from build123d import *

# Parameters (mm, degrees)
SKETCH_1_W               = 164.5
SKETCH_1_H               = 88.2
EXTRUDE_1_DEPTH          = 4
SKETCH_2_W               = 178.5
SKETCH_2_H               = 102.2
SKETCH_2_R               = 2.45
SKETCH_2_W_2             = 164.5
SKETCH_2_H_2             = 88.2
EXTRUDE_3_DEPTH          = 15
EXTRUDE_5_DEPTH          = 5
SKETCH_3_4_R             = 1.7
CUT_EXTRUDE_3_DEPTH      = 12
CUT_EXTRUDE_3_DEPTH_BACK = 5
EXTRUDE_6_DEPTH          = 5
SKETCH_4_3_R             = 1.4
CUT_EXTRUDE_4_DEPTH      = 12
CUT_EXTRUDE_4_DEPTH_BACK = 5
CUT_EXTRUDE_5_DEPTH      = 1
CUT_EXTRUDE_5_DEPTH_BACK = 179.5
CUT_EXTRUDE_6_DEPTH      = 2


with BuildPart() as part:
    # Sketch 1 → Extrude 1 (new body)
    with BuildSketch(Plane.XY):
        Rectangle(SKETCH_1_W, SKETCH_1_H)
    extrude(amount=EXTRUDE_1_DEPTH)

    # Sketch 2 → Extrude 3 (add)
    with BuildSketch(Plane.XY.offset(4)):
        Rectangle(SKETCH_2_W, SKETCH_2_H)
        with Locations((-85.75, 47.6)):
            Circle(SKETCH_2_R, mode=Mode.SUBTRACT)
        with Locations((-85.75, -47.6)):
            Circle(SKETCH_2_R, mode=Mode.SUBTRACT)
        with Locations((85.75, 47.6)):
            Circle(SKETCH_2_R, mode=Mode.SUBTRACT)
        with Locations((85.75, -47.6)):
            Circle(SKETCH_2_R, mode=Mode.SUBTRACT)
        Rectangle(SKETCH_2_W_2, SKETCH_2_H_2, mode=Mode.SUBTRACT)
    extrude(amount=-EXTRUDE_3_DEPTH)

    # Sketch 3 → Extrude 5 (add)
    with BuildSketch(Plane(origin=(0, 0, 0), x_dir=(-1, 0, 0), z_dir=(0, 0, -1))):
        Polygon((-21.7, 29.6), (-21.7, -29.7), (21.7, -29.7), (21.7, 29.6), (11, 29.6), (11, 27.1), (19.2, 27.1), (19.2, -27.2), (-19.2, -27.2), (-19.2, 27.1), (0, 27.1), (0, 29.6), align=None)
    extrude(amount=EXTRUDE_5_DEPTH)

    # Sketch 3_4 → Cut-Extrude 3 (cut, two sides)
    with BuildSketch(Plane(origin=(0, 0, 0), x_dir=(-1, 0, 0), z_dir=(0, 0, -1))) as cut_extrude_3_sk:
        with Locations((3.71, -24)):
            Circle(SKETCH_3_4_R)
        with Locations((10, 12.5)):
            Circle(SKETCH_3_4_R)
    extrude(amount=CUT_EXTRUDE_3_DEPTH, mode=Mode.SUBTRACT)
    extrude(cut_extrude_3_sk.sketch, amount=-CUT_EXTRUDE_3_DEPTH_BACK, mode=Mode.SUBTRACT)

    # Sketch 4 → Extrude 6 (add)
    with BuildSketch(Plane(origin=(0, 0, 0), x_dir=(-1, 0, 0), z_dir=(0, 0, -1))):
        Polygon((75.895357905, 39.183227458), (75.895357905, 14.983227458), (78.395357905, 14.983227458), (78.395357905, 41.683227458), (29.395357905, 41.683227458), (29.395357905, 14.983227458), (31.895357905, 14.983227458), (31.895357905, 39.183227458), align=None)
        Polygon((-77.674472702, 40.885349978), (-28.674472702, 40.885349978), (-28.674472702, 14.185349978), (-31.174472702, 14.185349978), (-31.174472702, 38.385349978), (-75.174472702, 38.385349978), (-75.174472702, 14.185349978), (-77.674472702, 14.185349978), align=None)
    extrude(amount=EXTRUDE_6_DEPTH)

    # Sketch 4_3 → Cut-Extrude 4 (cut, two sides)
    with BuildSketch(Plane(origin=(0, 0, 0), x_dir=(-1, 0, 0), z_dir=(0, 0, -1))) as cut_extrude_4_sk:
        with Locations((72.695357905, 35.983227458)):
            Circle(SKETCH_4_3_R)
        with Locations((72.695357905, -1.616772542)):
            Circle(SKETCH_4_3_R)
        with Locations((35.095357905, -1.616772542)):
            Circle(SKETCH_4_3_R)
        with Locations((35.095357905, 35.983227458)):
            Circle(SKETCH_4_3_R)
        with Locations((-34.374472702, 35.185349978)):
            Circle(SKETCH_4_3_R)
        with Locations((-34.374472702, -2.414650022)):
            Circle(SKETCH_4_3_R)
        with Locations((-71.974472702, -2.414650022)):
            Circle(SKETCH_4_3_R)
        with Locations((-71.974472702, 35.185349978)):
            Circle(SKETCH_4_3_R)
    extrude(amount=CUT_EXTRUDE_4_DEPTH, mode=Mode.SUBTRACT)
    extrude(cut_extrude_4_sk.sketch, amount=-CUT_EXTRUDE_4_DEPTH_BACK, mode=Mode.SUBTRACT)

    # Sketch 5 → Cut-Extrude 5 (cut, two sides)
    with BuildSketch(Plane.ZY.offset(89.25)) as cut_extrude_5_sk:
        Polygon((-8.55, -20.3), (-5.75, -20.3), (-3, -23.5), (-3, -36.1), (-11.3, -36.1), (-11.3, -23.5), align=None)
    extrude(amount=CUT_EXTRUDE_5_DEPTH, mode=Mode.SUBTRACT)
    extrude(cut_extrude_5_sk.sketch, amount=-CUT_EXTRUDE_5_DEPTH_BACK, mode=Mode.SUBTRACT)

    # Sketch 6 → Cut-Extrude 6 (cut)
    with BuildSketch(Plane.XY.offset(4)):
        Polygon((-37.866270853, 36.028409728), (-36.519943372, 33.606137589), (-33.749030425, 33.560955319), (-32.324444958, 35.938045189), (-33.670772438, 38.360317328), (-36.441685386, 38.405499597), align=None)
        Polygon((-71.349030425, 33.560955319), (-69.924444958, 35.938045189), (-71.270772438, 38.360317328), (-74.041685386, 38.405499597), (-75.466270853, 36.028409728), (-74.119943372, 33.606137589), align=None)
        Polygon((-33.670772438, 0.760317328), (-36.441685386, 0.805499597), (-37.866270853, -1.571590272), (-36.519943372, -3.993862411), (-33.749030425, -4.039044681), (-32.324444958, -1.661954811), align=None)
        Polygon((-71.349030425, -4.039044681), (-69.924444958, -1.661954811), (-71.270772438, 0.760317328), (-74.041685386, 0.805499597), (-75.466270853, -1.571590272), (-74.119943372, -3.993862411), align=None)
        Polygon((35.799058169, 37.562439847), (33.028145222, 37.607622117), (31.603559755, 35.230532247), (32.949887235, 32.808260108), (35.720800183, 32.763077839), (37.14538565, 35.140167708), align=None)
        Polygon((33.028145222, 0.007622117), (31.603559755, -2.369467753), (32.949887235, -4.791739892), (35.720800183, -4.836922161), (37.14538565, -2.459832292), (35.799058169, -0.037560153), align=None)
        Polygon((69.203559755, 35.230532247), (70.549887235, 32.808260108), (73.320800183, 32.763077839), (74.74538565, 35.140167708), (73.399058169, 37.562439847), (70.628145222, 37.607622117), align=None)
        Polygon((73.399058169, -0.037560153), (70.628145222, 0.007622117), (69.203559755, -2.369467753), (70.549887235, -4.791739892), (73.320800183, -4.836922161), (74.74538565, -2.459832292), align=None)
        Polygon((-11.346327481, 14.922272139), (-12.770912947, 12.54518227), (-11.424585467, 10.122910131), (-8.653672519, 10.077727861), (-7.229087053, 12.45481773), (-8.575414533, 14.877089869), align=None)
        Polygon((-5.056327481, -21.577727861), (-6.480912947, -23.95481773), (-5.134585467, -26.377089869), (-2.363672519, -26.422272139), (-0.939087053, -24.04518227), (-2.285414533, -21.622910131), align=None)
    extrude(amount=-CUT_EXTRUDE_6_DEPTH, mode=Mode.SUBTRACT)


solid = part.part
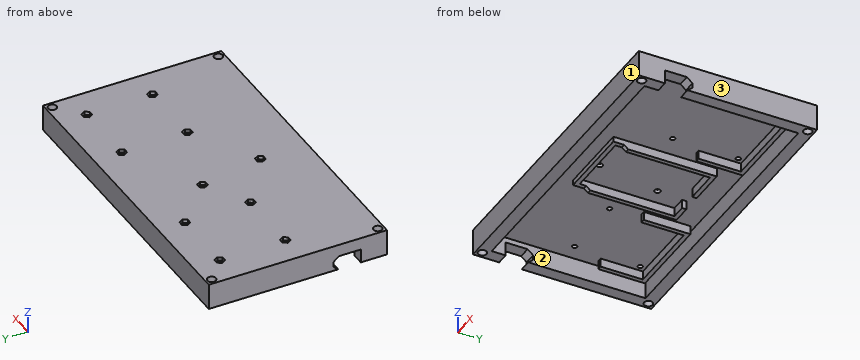
Source: CAD feature listing. Evaluate the final solid. Frame: model axes, mm. Face numbers are marked on the shaded views. Give positions to 0.01 mm unless a question says otherwise; leave off trailing zeros. Write each loop counter-clockwise with the first axis right and the second up, starting at its lowest first coordinate (ties: lowest second). Pieces come first, ordered by that corner, then holes. Notation, with made-up numbers: (73.5, 69.25) -> (83.5, 69.25) arc R8 cw to (83.5, 77.25) -> close; hole circle Ø7 at (51.25, -13). An arc over 180 degrees is marked (long way). Write item = value, one per line.
Q1. Cut plane A-A on x = 85.75. Return loops of the section in (y, z), then the cut area to 3 significant figures.
Here are the results:
outline = (-51.1, -11) -> (-50.05, -11) -> (-50.05, 4) -> (-51.1, 4) -> close; (-45.15, -11) -> (-36.1, -11) -> (-36.1, -3) -> (-23.5, -3) -> (-20.3, -5.75) -> (-20.3, -8.55) -> (-23.15, -11) -> (45.15, -11) -> (45.15, 4) -> (-45.15, 4) -> close; (50.05, -11) -> (51.1, -11) -> (51.1, 4) -> (50.05, 4) -> close
area = 1,270 mm²
Q2. Cut plane C-C on x = 41.5. Return loops of the section in (y, z), then the cut area to 3 significant figures.
Here are the results:
outline = (-51.1, -11) -> (-44.1, -11) -> (-44.1, 0) -> (38.39, 0) -> (38.39, -5) -> (40.89, -5) -> (40.89, 0) -> (44.1, 0) -> (44.1, -11) -> (51.1, -11) -> (51.1, 4) -> (-51.1, 4) -> close
area = 575 mm²
Q3. First-contact query: pin 1 (2 mm diameter, centred on x = 49, y = -19.5, fed in from -Z); pin 2 (5 mm diameter, centred on x = -70, y = 38, fed in from -Z). Flat tips, straight axial feed; report the tip coordinate or a pass-through.
Here are the results:
pin_1 = 0
pin_2 = -5
Q4. Mould query, pull axis X, two halves, no side actions, for the marked faces 1, 2 and 3. Classes: +X half, -X half, draft (parallel to the pull), parting line (faces both ways), or undercut.
Here are the results:
face_1 = draft
face_2 = undercut
face_3 = +X half
Q5. Line query: line 1 (X direction, y = 9.5, z = -4.5); line 2 (Y direction, x = -73.5, z = -3); line 3 (X direction, y = 25, z = -6.75). Output: solid intervals per line, ascending. Write a range as from..to.
Here are the results:
line_1 = -89.25..-82.25, -21.7..-19.2, 19.2..21.7, 82.25..89.25
line_2 = -51.1..-44.1, 39.18..41.68, 44.1..51.1
line_3 = -89.25..-82.25, 82.25..89.25
Q6. Cut plane B-B on y = -47.6. Return loops of the section in (x, z), then the cut area to 3 significant figures.
Here are the results:
outline = (-89.25, -11) -> (-88.2, -11) -> (-88.2, 4) -> (-89.25, 4) -> close; (-83.3, -11) -> (83.3, -11) -> (83.3, 4) -> (-83.3, 4) -> close; (88.2, -11) -> (89.25, -11) -> (89.25, 4) -> (88.2, 4) -> close
area = 2,530 mm²
